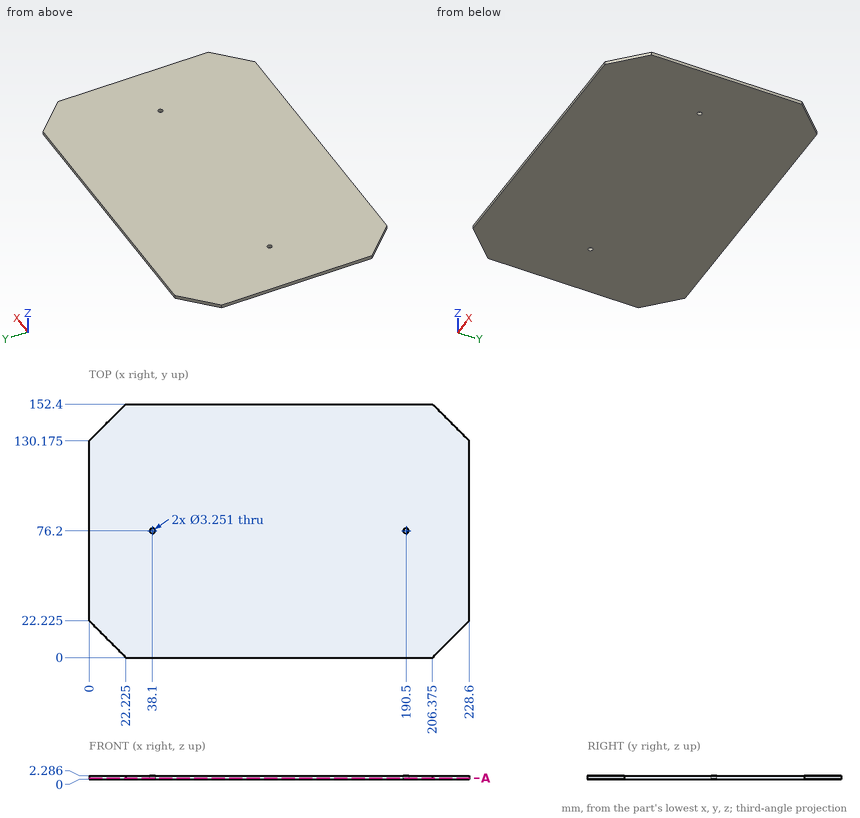
Study the drawing (mm; zero at the part's minimum x, y, z) and answer. Give positions to 0.01 mm unless a question says otherwise; leave off trailing zeros. Loops run counter-clockwise (first coordinate to the right, second up) from the corner with the lowest first, then second, coordinate; pieces in that order, holes last. Notation, with made-up numbers: M 29,14.5 L 75,14.5 A18 cw 75,41.5 Z; hole C 42.25,52 d10. An arc over 180 degrees is marked long. One line per item, written item: value.
1. Section A-A on z = 0.75 is taken. Determine the outline of the cut face in (x, y) (1 decimal).
Found:
outline: M 0,22.2 L 22.2,0 L 206.4,0 L 228.6,22.2 L 228.6,130.2 L 206.4,152.4 L 22.2,152.4 L 0,130.2 Z; hole C 38.1,76.2 d3.3; hole C 190.5,76.2 d3.3
2. This flat-tipped pin is pushed along its axis until it touches: P1, Ø2.5, axis at x = 38.1, y = 76.2, coming from the -Z side. Where does it stop, or does it pass through?
Found:
P1: through
3. Find the intervals of material crossed by probe 1 along X at (y, z) = (76.2, 1.75); probe 2 along Y at (x, z) = (38.1, 0.9); probe 3 along Y at (x, z) = (212.5, 1.1) (1 decimal), in increasing order.
Found:
probe 1: 0 to 36.47, 39.73 to 188.87, 192.13 to 228.6
probe 2: 0 to 74.57, 77.83 to 152.4
probe 3: 6.1 to 146.3
